Autodesk Inventor part; units mm, degrees
ref_plane "Startebene" through (0, 0, 0) normal (0, 0, 1) x (1, 0, 0)
ref_plane "Endebene" through (0, 0, 120) normal (0, 0, 1) x (1, 0, 0)
ref_plane "YZ Plane" through (0, 0, 0) normal (1, 0, 0) x (0, 1, 0)
ref_plane "Startebene" through (0, 0, 0) normal (0, 0, 1) x (1, 0, 0)
ref_plane "Endebene" through (0, 0, 120) normal (0, 0, 1) x (1, 0, 0)
sketch "Skizze" plane through (0, 0, 0) normal (0, 0, 1) x (1, 0, 0)
  line L0 (4, -30) -> (-4, -30)
  line L1 (-4, -30) -> (-4, 30)
  line L2 (-4, 30) -> (4, 30)
  line L3 (4, 30) -> (4, -30)
  line L4 (-6, 0) -> (8, 0) construction
  line L5 (0, -30) -> (0, 40) construction
  line L6 (0, 54) -> (0, -44) construction
  line L7 (-9.2, 0) -> (13.2, 0) construction
  dimension "d0" = 60
  dimension "d1" = 8
  dimension "d4" = 4
  dimension "d5" = 30
extrude "Körper" add sketch "Skizze" along normal up to surface (120 mm away) from surface at 0
sketch "Sketch3" plane through (0, 0, 0) normal (0, 0, 1) x (1, 0, 0)
  line L0 (0, 0) -> (10, 0)
ref_plane "Work Plane3" through (0, 0, 0) normal (0, -1, 0) x (1, 0, 0)
sketch "Sketch4" plane through (0, 0, 0) normal (0, -1, 0) x (1, 0, 0)
  line L0 (-2, 0) -> (12, 0)
  line L1 (-2, 120) -> (12, 120)
  dimension "d9" = 120
sketch "Skizze5" plane through (4, -30, 120) normal (1, 0, 0) x (0, 0, -1)
  line L0 (0, 60) -> (0, 0)
  line L1 (120, 0) -> (0, 0)
  line L2 (0, 60) -> (0, 0)
  line L3 (120, 0) -> (0, 0)
  line L4 (120, 60) -> (120, 0)
  line L5 (120, 60) -> (0, 60)
  point P0 (120, 30)
  point P1 (30, 30)
  dimension "d10" = 30
  dimension "d11" = 30
hole "Bohrung1" at (4, 0, 90) direction (-1, 0, 0) diameter 16 end through all
sketch "Skizze6" plane through (4, -30, 120) normal (1, 0, 0) x (0, 0, -1)
  circle A0 centre (30, 30) radius 8
  line L0 (120, 60) -> (0, 60)
  line L1 (0, 0) -> (60, 0)
  line L2 (60, 0) -> (60, 60)
  line L3 (60, 60) -> (0, 60)
  line L4 (0, 60) -> (0, 0)
  point P0 (120, 30)
  dimension "d19" = 60
extrude "Extrusion2" cut sketch "Skizze6" against normal blind 1
sketch "Skizze7" plane through (-4, 30, 0) normal (-1, 0, 0) x (0, 0, 1)
  circle A0 centre (90, -30) radius 8
  line L0 (120, -60) -> (60, -60)
  line L1 (60, -60) -> (60, 0.4696)
  line L2 (60, 0.4696) -> (120, 0.4696)
  line L3 (120, 0.4696) -> (120, -60)
  point P0 (0, -30)
  dimension "d22" = 60
extrude "Extrusion3" cut sketch "Skizze7" against normal blind 1
equation "\"d0\" = G_W"
equation "\"d1\" = G_H"
equation "\"d4\" = 0.5 * d1"
equation "\"d5\" = 0.5 * d0"
equation "\"d2\" = G_L"
equation "\"G_W\" = 60"
equation "\"G_H\" = 8"
equation "\"G_L\" = d9"
equation "\"G_OFFSET_START\" = 0"
equation "\"G_OFFSET_END\" = 0"
properties part number "EN 10058 - 60 x 8 - 110" material "Stahl, weich"
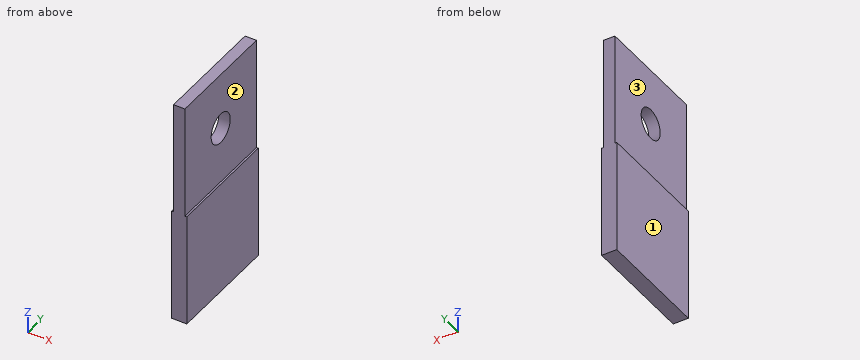
Could you check a few things on this model? Use its own coordinates, in mm. Face numbers are marked on the shaded views. A direction names the side the tool comes from. Coordinates: 2 decimals unless noted, no trailing zeros. Write each loop counter-clockwise with the first axis right and the second up, starting at its lowest first coordinate (ties: lowest second). Pieces come first, ordered by that corner, then holes. Notation, with made-up numbers: (-9, 28) -> (38, 28) arc R14 cw to (38, 55) -> close; hole circle Ø9 at (57, 54). An arc over 180 degrees is marked (long way). One line per question, with ' | ' between items. Start each with the question number.
1. If we section it at A-A (y = 0): Please give me the cut outline in (x, z), and give its area (3 significant figures).
2. If we section it at D-D (y = -18.5): Please give me the cut outline in (x, z), and give its area (3 significant figures).
3. For the marked faces 1, 2 and 3, which set-ups out of +Z, -Z, +X, -X, +Y, -Y let a thin tool reach every point of the face, with its end or its side?
4. If we section it at C-C (x = 1.75): Please give me the cut outline in (y, z).
5. If we section it at B-B (z = 90): Please give me the cut outline in (x, y), and give its area (3 significant figures).
6. Will these pins go through, and if not, where does the flat tip stop? P1, Ø0.5, axis at x = 3.5, y = 1.5, coming from the +Z side; P2, Ø2, axis at y = -20.5, z = 93, coming from the -X side; P3, Ø4, axis at y = 23.5, z = 67.5, coming from the +X side.
7. Please list where these lines run through material, in increasing order: line 1 along Y through (x, z) = (0.8, 90); line 2 along Z through (x, y) = (3.5, -4); line 3 along X through (y, z) = (-3.5, 71.5).
Return value:
1) outline: (-4, 0) -> (4, 0) -> (4, 60) -> (3, 60) -> (3, 82) -> (-3, 82) -> (-3, 60) -> (-4, 60) -> close; (-3, 98) -> (3, 98) -> (3, 120) -> (-3, 120) -> close | area: 744 mm²
2) outline: (-4, 0) -> (4, 0) -> (4, 60) -> (3, 60) -> (3, 120) -> (-3, 120) -> (-3, 60) -> (-4, 60) -> close | area: 840 mm²
3) face 1: +Z, -Z, -X, +Y, -Y | face 2: +Z, +X, +Y, -Y | face 3: +Z, -X, +Y, -Y
4) outline: (-30, 0) -> (30, 0) -> (30, 120) -> (-30, 120) -> close; hole circle Ø16 at (0, 90)
5) outline: (-3, -30) -> (3, -30) -> (3, -8) -> (-3, -8) -> close; (-3, 8) -> (3, 8) -> (3, 30) -> (-3, 30) -> close | area: 264 mm²
6) P1: stops at z = 60 | P2: stops at x = -3 | P3: stops at x = 3
7) line 1: y = -30 to -8, 8 to 30 | line 2: z = 0 to 60 | line 3: x = -3 to 3
